Work out the finished part from the listing and answer in its coordinate system (mm). A direction names the side the tool comes from. Coordinates: 2 decimals unless noted, no trailing zeros. Write each loop counter-clockwise with the first axis right and the second up, starting at its lowest first coordinate (ties: lowest second). Pieces come first, ordered by that corner, then holes. Notation, with made-up numbers: (-24.5, 52.25) - (-20.5, 52.25) arc R10 cw to (-20.5, 65.25) - close; hole circle Ø11 at (58.25, 2.5). An arc over 180 degrees is marked (long way). One line per item, written item: value.
```python
from build123d import *

# Parameters (mm, degrees)
SKETCH001_W      = 18
SKETCH001_H      = 2.4
EXTRUDE001_DEPTH = 5
SKETCH_W         = 23.8
SKETCH_H         = 10.2
EXTRUDE_DEPTH    = 10


with BuildPart() as extrude001:
    # Sketch001 (on Face6 of Extrude) → Extrude001 (new body)
    with BuildSketch(Plane.XY.offset(10)):
        Rectangle(SKETCH001_W, SKETCH001_H)
    extrude(amount=-EXTRUDE001_DEPTH)


with BuildPart() as cut:
    # Sketch → Extrude (new body)
    with BuildSketch(Plane.XY):
        Rectangle(SKETCH_W, SKETCH_H)
    extrude(amount=EXTRUDE_DEPTH)

    # Cut: cut Extrude001
    add(extrude001.part, mode=Mode.SUBTRACT)


solid = cut.part
```
Item 1: Section B-B, the plane y = 0 is taken. Determine the outline of the cut face in (x, z), then the cut area to 3 significant figures.
Evaluation:
outline: (-11.9, 0) - (11.9, 0) - (11.9, 10) - (9, 10) - (9, 5) - (-9, 5) - (-9, 10) - (-11.9, 10) - close
area: 148 mm2
Item 2: Consider probe 1 along Y at (x, z) = (-5.75, 8.5); probe 2 along X at (y, z) = (-0.75, 7); probe 3 along Z at (x, y) = (-2.5, -0.5). Determine where each line is inside the solid, lowest interval first.
Evaluation:
probe 1: y = -5.1 to -1.2, 1.2 to 5.1
probe 2: x = -11.9 to -9, 9 to 11.9
probe 3: z = 0 to 5
Item 3: Given pin 1 (2 mm diameter, centred on x = -7.5, y = -1.5, fed in from -Z); pin 2 (1.9 mm diameter, centred on x = 1, y = 0, fed in from +Z), each flat-ended and moving along its own axis, determine where each tip first touches the part or whether it passes through.
Evaluation:
pin 1: stops at z = 0
pin 2: stops at z = 5
Item 4: Determine the mould class of faces 1 (the face through (11.9, 0, 5)), 2 (the face through (-11.9, 0, 5)), 3 (the face through (0, 1.2, 8)), 4 (the face through (0, 2, 10)) for opening direction X: +X half, -X half, draft (parallel to the pull), parting line (faces both ways), or undercut.
Evaluation:
face 1: +X half
face 2: -X half
face 3: undercut
face 4: draft
Item 5: Section A-A, the plane z = 6.5 is taken. Determine the outline of the cut face in (x, y), then the cut area to 3 significant figures.
Evaluation:
outline: (-11.9, -5.1) - (11.9, -5.1) - (11.9, 5.1) - (-11.9, 5.1) - close; hole (-9, -1.2) - (9, -1.2) - (9, 1.2) - (-9, 1.2) - close
area: 200 mm2
Item 6: Which of the six approach directions +Z, -Z, +X, -X, +Y, -Y give full straight-line access (tool end or side, diameter ignored) to faces 5 (the face through (-9, 0, 8)), 6 (the face through (0, -5.1, 5))?
Evaluation:
face 5: +Z
face 6: +Z, -Z, +X, -X, -Y
Item 7: Section C-C, the plane x = -1.5 is taken. Determine the outline of the cut face in (y, z).
Evaluation:
outline: (-5.1, 0) - (5.1, 0) - (5.1, 10) - (1.2, 10) - (1.2, 5) - (-1.2, 5) - (-1.2, 10) - (-5.1, 10) - close
